Work out the finished part from the listing and answer in its coordinate system (mm). A direction names the side the tool comes from. Round coordinates to 2 decimals unless told otherwise and drop trailing zeros. Write each loop counter-clockwise with the first axis right and the second up, starting at its lowest first coordinate (ties: lowest second). Pieces come first, ordered by that corner, then holes. Notation, with made-up numbers: (-35, -24) -> (-19, -24) arc R23 ccw to (-19, 7) -> close; hole circle Ø10 at (-29.75, 63). An arc over 180 degrees is marked (long way). Answer as a JSON object with one key per item and string values. Group by question number.
from build123d import *

# Parameters (mm, degrees)
SKETCH1_W           = 24.7
SKETCH1_H           = 24.7
BOSS_EXTRUDE1_DEPTH = 200
SKETCH1_4_W         = 12
SKETCH1_4_H         = 12
CUT_EXTRUDE1_DEPTH  = 193.65
SKETCH2_R           = 3.175
CUT_EXTRUDE2_DEPTH  = 203.353187521


with BuildPart() as part:
    # Sketch1 → Boss-Extrude1 (new body)
    with BuildSketch(Plane.XY):
        with Locations((6, 6)):
            Rectangle(SKETCH1_W, SKETCH1_H)
    extrude(amount=BOSS_EXTRUDE1_DEPTH)

    # Sketch1<4> → Cut-Extrude1 (cut)
    with BuildSketch(Plane.XY):
        with Locations((6, 6)):
            Rectangle(SKETCH1_4_W, SKETCH1_4_H)
    extrude(amount=CUT_EXTRUDE1_DEPTH, mode=Mode.SUBTRACT)

    # Sketch2 → Cut-Extrude2 (cut, through all)
    with BuildSketch(Plane(origin=(0, 18.35, 0), x_dir=(1, 0, 0), z_dir=(0, 1, 0))):
        with Locations(Location((6, -184.76, 0), (0, 0, 270))):
            Circle(SKETCH2_R)
    extrude(amount=-CUT_EXTRUDE2_DEPTH, mode=Mode.SUBTRACT)


solid = part.part
1) A cutting plane is placed at A-A on x = 6. Determine the outline of the cut face in (y, z) (3 decimals).
2) A cutting plane is placed at B-B on z = 184.76. Determine the outline of the cut face in (x, y) (3 decimals), plus the area to 3 significant figures.
3) A cutting plane is placed at D-D on z = 143. Determine the outline of the cut face in (x, y), plus the area to 3 significant figures.
4) A tool of negligible diameter and unlimited length cuts with its end or side. For faces 1 (the face through (6.14, 15.22, 181.59)), 2 (the face through (12, 6, 95)), from which of +Z, -Z, +X, -X, +Y, -Y can it reach the whole face along a straight path? Write none if from no direction.
5) For a pull along X with two mould halves and no side action, classify faces 3 (the face through (6, 6, 200)), 4 (the face through (0, 6, 95)), 5 (the face through (18.35, 6, 99)) as released by +X, released by -X, zero draft, split by the parting line, or undercut.
6) This flat-tipped pin is pushed along its axis until it touches: P1, Ø3.5, axis at x = 3.5, y = 4.5, coming from the -Z side. Where does it stop, or does it pass through?
7) A cutting plane is placed at C-C on y = 6.5. Determine the outline of the cut face in (x, z), plus the area to 3 significant figures.
8) Straight lines are drawn through the part: L1, parallel to Y at x = 6, z = 177; L2, parallel to X at y = 16.75, z = 184.76 (3 decimals). For each, find the intervals that lie inside material, in ascending order.
Established:
{
 "1": {"outline": "(-6.35, 0) -> (0, 0) -> (0, 181.585) -> (-6.35, 181.585) -> close; (-6.35, 187.935) -> (0, 187.935) -> (0, 193.65) -> (12, 193.65) -> (12, 187.935) -> (18.35, 187.935) -> (18.35, 200) -> (-6.35, 200) -> close; (12, 0) -> (18.35, 0) -> (18.35, 181.585) -> (12, 181.585) -> close"},
 "2": {"outline": "(-6.35, -6.35) -> (2.825, -6.35) -> (2.825, 0) -> (0, 0) -> (0, 12) -> (2.825, 12) -> (2.825, 18.35) -> (-6.35, 18.35) -> close; (9.175, -6.35) -> (18.35, -6.35) -> (18.35, 18.35) -> (9.175, 18.35) -> (9.175, 12) -> (12, 12) -> (12, 0) -> (9.175, 0) -> close", "area": "385 mm²"},
 "3": {"outline": "(-6.35, -6.35) -> (18.35, -6.35) -> (18.35, 18.35) -> (-6.35, 18.35) -> close; hole (0, 0) -> (12, 0) -> (12, 12) -> (0, 12) -> close", "area": "466 mm²"},
 "4": {"face 1": "+Y, -Y", "face 2": "-Z"},
 "5": {"face 3": "zero draft", "face 4": "undercut", "face 5": "released by +X"},
 "6": {"P1": "stops at z = 193.65"},
 "7": {"outline": "(-6.35, 0) -> (0, 0) -> (0, 193.65) -> (12, 193.65) -> (12, 0) -> (18.35, 0) -> (18.35, 200) -> (-6.35, 200) -> close", "area": "2,620 mm²"},
 "8": {"L1": "y = -6.35 to 0, 12 to 18.35", "L2": "x = -6.35 to 2.825, 9.175 to 18.35"}
}
